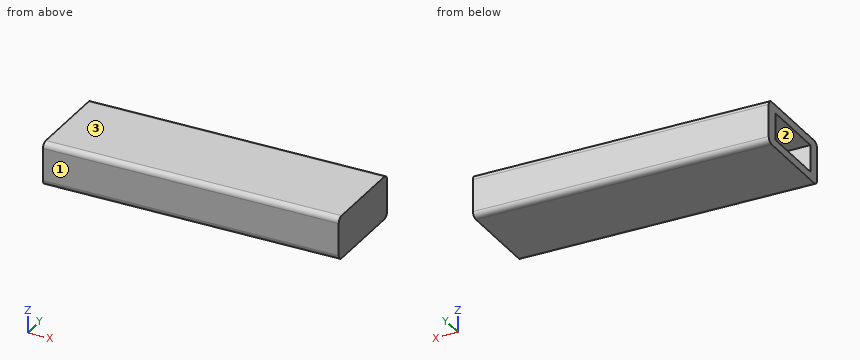
```python
from build123d import *

# Parameters (mm, degrees)
F2_DEPTH = 55
F3_W     = 12.4
F3_H     = 5
F4_DEPTH = 14
F6_ANGLE = 90


with BuildPart() as f2:
    # F1 (on face) → F2 (new body)
    with BuildSketch(Plane.XZ):
        with BuildLine():
            Line((7.5, 4), (-7.5, 4))
            ThreePointArc((-7.5, 4), (-8.2071067812, 3.7071067812), (-8.5, 3))
            Line((-8.5, 3), (-8.5, -3))
            ThreePointArc((-8.5, -3), (-8.2071067812, -3.7071067812), (-7.5, -4))
            Line((-7.5, -4), (7.5, -4))
            ThreePointArc((7.5, -4), (8.2071067812, -3.7071067812), (8.5, -3))
            Line((8.5, -3), (8.5, 3))
            ThreePointArc((8.5, 3), (8.2071067812, 3.7071067812), (7.5, 4))
        make_face()
    extrude(amount=F2_DEPTH)

    # F3 (on face) → F4 (cut)
    with BuildSketch(Plane.XZ.offset(55)):
        Rectangle(F3_W, F3_H)
    extrude(amount=-F4_DEPTH, mode=Mode.SUBTRACT)


with BuildPart() as f2_1:
    # F6: moved
    add(f2.part.rotate(Axis((-8.5, -55, 0), (0, 0, -1)), F6_ANGLE))


solid = f2_1.part
```
Could you check a few things on this model? Use its own coordinates, in mm. Face numbers are marked on the shaded views. Coordinates: 2 decimals unless noted, no trailing zeros. Order: outer loops, then holes, each group sorted by start corner. A loop starts at its lowest first (then second) coordinate and runs counter-clockwise, first axis right, second up. Notation, with made-up numbers: M 15.5,57.25 L 66.5,57.25 A22 ccw 66.5,76.25 Z; hole C -29,89.25 d3. An arc over 180 degrees is marked long. Use a Markdown table: item, result. Add a question column.
Q1. I want a section at C-C on z = -1.5. List the corners of the cut face in (x, y) for me, then the cut area to 3 significant figures.
Q2. We'd pull the mould along Y, two halves only. Please class the marked faces 1, 2 and 3: pulls with the +Y half, pulls with the -Y half, needs draft (parallel to the pull), parting line crosses it, or undercut.
Q3. I want a section at A-A on y = -66.25. List the corners of the cut face in (x, z) for me.
Q4. I'm going to push a flat-ended pin straight in: pin 1 (2.5 mm diameter, centred on y = -66.5, z = -0.5, fed in from -X). Where does the tip first touch, or does it pass through?
Q5. I want a section at B-B on x = -4.5. List the corners of the cut face in (y, z) for me.
Q6. If I drill on L1, parallel to Z at x = -1.5, y = -69.5; L2, parallel to X at y = -66.5, z = 0.25; L3, parallel to Y at x = -2, z = 1.25, over which ranges is the centre line in solid material (lowest first)?
Checked values:
| question | item | result |
|---|---|---|
| 1 | outline | M -8.5,-72 L 46.5,-72 L 46.5,-55 L -8.5,-55 L -8.5,-57.3 L 5.5,-57.3 L 5.5,-69.7 L -8.5,-69.7 Z |
| 1 | area | 761 mm² |
| 2 | face 1 | pulls with the -Y half |
| 2 | face 2 | undercut |
| 2 | face 3 | needs draft |
| 3 | outline | M -8.5,-4 L 46.5,-4 L 46.5,4 L -8.5,4 L -8.5,2.5 L 5.5,2.5 L 5.5,-2.5 L -8.5,-2.5 Z |
| 4 | pin 1 | x = 5.5 |
| 5 | outline | M -72,-3 A1 ccw -71,-4 L -56,-4 A1 ccw -55,-3 L -55,3 A1 ccw -56,4 L -71,4 A1 ccw -72,3 Z; hole M -69.7,-2.5 L -57.3,-2.5 L -57.3,2.5 L -69.7,2.5 Z |
| 6 | L1 | -4 to -2.5, 2.5 to 4 |
| 6 | L2 | 5.5 to 46.5 |
| 6 | L3 | -72 to -69.7, -57.3 to -55 |
